```python
from build123d import *

# Parameters (mm, degrees)
SKETCH_1_R            = 7
EXTRUDE_1_DEPTH       = 10
SKETCH_9_W            = 7.120641766
SKETCH_9_H            = 4.534999238
EXTRUDE_6_DEPTH       = 1
SKETCH_11_W           = 1.257653538
SKETCH_11_H           = 9
EXTRUDE_7_DEPTH       = 4.5
EXTRUDE_8_DEPTH       = 6
FILLET_8_R            = 1
FILLET_9_R            = 1
CUT_EXTRUDE_1_DEPTH   = 10
SKETCH_14_W           = 1
SKETCH_14_H           = 3
EXTRUDE_9_DEPTH       = 3.122043073
SKETCH_15_W           = 1
SKETCH_15_H           = 3
EXTRUDE_10_DEPTH      = 4
EXTRUDE_11_DEPTH      = 0.2
EXTRUDE_11_DEPTH_BACK = 1.043632387
SKETCH_16_W           = 9.952294967
SKETCH_16_H           = 3.01746433
FILLET_11_R           = 1
FILLET_12_R           = 1
FILLET_13_R           = 1
FILLET_14_R           = 1
CUT_EXTRUDE_2_DEPTH   = 10
SKETCH_18_W           = 2.5
SKETCH_18_H           = 7.68123899
CUT_EXTRUDE_3_DEPTH   = 10
SKETCH_19_W           = 1.790352256
SKETCH_19_H           = 7.68123899
CUT_EXTRUDE_4_DEPTH   = 2
SKETCH_20_W           = 1.790352256
SKETCH_20_H           = 7.649055087
CUT_EXTRUDE_5_DEPTH   = 2
FILLET_15_R           = 1
FILLET_16_R           = 1
FILLET_17_R           = 1
FILLET_18_R           = 1


with BuildPart() as part:
    # Sketch 1 → Extrude 1 (new body)
    with BuildSketch(Plane(origin=(0.382706605, 0, 0), x_dir=(1, 0, 0), z_dir=(0, 0, 1))):
        with Locations((-75.594417438, 2.55)):
            Circle(SKETCH_1_R)
    extrude(amount=EXTRUDE_1_DEPTH)

    # Sketch 9 → Extrude 6 (add)
    with BuildSketch(Plane(origin=(6.127831546, 0, 9), x_dir=(1, 0, 0), z_dir=(0, 0, 1))):
        with Locations((-75.644850643, 2.267499619)):
            Rectangle(SKETCH_9_W, SKETCH_9_H)
    extrude(amount=EXTRUDE_6_DEPTH)



with BuildPart() as body_2:
    # Sketch 11 → Extrude 7 (new body)
    with BuildSketch(Plane(origin=(9.574526933, 4.534999238, 0.48426017), x_dir=(1, 0, 0), z_dir=(0, 1, 0))):
        with Locations((-76.184774061, -4.5)):
            Rectangle(SKETCH_11_W, SKETCH_11_H)
    extrude(amount=-EXTRUDE_7_DEPTH)


with BuildPart() as part_1:
    add(part.part)

    add(body_2.part)  # Extrude 8 merges body 2
    # Sketch 12 → Extrude 8 (add)
    with BuildSketch(Plane.ZY.offset(67.239073897)):
        Polygon((0.48426017, 4.534999238), (0.48426017, 0), (1.483647509, 0.034999238), (1.483647509, 4.534999238), align=None)
    extrude(amount=EXTRUDE_8_DEPTH)

    # Fillet 8
    fillet_8_edges = [part_1.edges().sort_by_distance(p)[0] for p in [
        (-65.981420359, 2.284999238, 0.48426017),
    ]]
    fillet(fillet_8_edges, radius=FILLET_8_R)

    # Fillet 9
    fillet_9_edges = [part_1.edges().sort_by_distance(p)[0] for p in [
        (-65.956698214, 2.267499619, 10),
    ]]
    fillet(fillet_9_edges, radius=FILLET_9_R - 0.0001)  # a hair under: the kernel refuses the full size

    # Sketch 13 → Cut-Extrude 1 (cut)
    with BuildSketch(Plane(origin=(0, 0, 0), x_dir=(-1, 0, 0), z_dir=(0, 0, -1))):
        with BuildLine():
            Line((69.812827514, 7.005564937), (69.812827514, -1.905564937))
            ThreePointArc((69.812827514, -1.905564937), (67.081734981, 2.55), (69.812827514, 7.005564937))
        make_face()
    extrude(amount=-CUT_EXTRUDE_1_DEPTH, mode=Mode.SUBTRACT)


with BuildPart() as cut_extrude_1_kept_piece:
    # of the separate pieces the step leaves, the one the design keeps (cut_extrude_1_pieces_kept)
    add(part_1.part.solids().sort_by_distance((-69.812827514, 7.005564937, 10))[0])

    # Sketch 14 → Extrude 9 (add)
    with BuildSketch(Plane(origin=(-69.812827514, 0, 0), x_dir=(0, 0, -1), z_dir=(1, 0, 0))):
        with Locations((-9.5, 2.417510407)):
            Rectangle(SKETCH_14_W, SKETCH_14_H)
    extrude(amount=EXTRUDE_9_DEPTH)

    # Sketch 15 → Extrude 10 (add)
    with BuildSketch(Plane(origin=(-69.812827514, 0, 0), x_dir=(0, 0, -1), z_dir=(1, 0, 0))):
        with Locations((-0.5, 2.417510407)):
            Rectangle(SKETCH_15_W, SKETCH_15_H)
    extrude(amount=EXTRUDE_10_DEPTH)

    # Sketch 16 → Extrude 11 (add, two sides: drawn at the far end of the back side and taken through both)
    with BuildSketch(Plane(origin=(-65.812827514, 0, 0), x_dir=(0, 0, -1), z_dir=(1, 0, 0)).offset(-EXTRUDE_11_DEPTH_BACK)):
        with Locations((-4.976147484, 2.408778242)):
            Rectangle(SKETCH_16_W, SKETCH_16_H)
    extrude(amount=EXTRUDE_11_DEPTH + EXTRUDE_11_DEPTH_BACK)

    # Fillet 11
    fillet_11_edges = [cut_extrude_1_kept_piece.edges().sort_by_distance(p)[0] for p in [
        (-65.612827514, 2.408778242, 0),
    ]]
    fillet(fillet_11_edges, radius=FILLET_11_R)

    # Fillet 12
    fillet_12_edges = [cut_extrude_1_kept_piece.edges().sort_by_distance(p)[0] for p in [
        (-65.612827514, 2.408778242, 9.952294967),
    ]]
    fillet(fillet_12_edges, radius=FILLET_12_R)

    # Fillet 13
    fillet_13_edges = [cut_extrude_1_kept_piece.edges().sort_by_distance(p)[0] for p in [
        (-69.812827514, 7.005564937, 5),
    ]]
    fillet(fillet_13_edges, radius=FILLET_13_R)

    # Fillet 14
    fillet_14_edges = [cut_extrude_1_kept_piece.edges().sort_by_distance(p)[0] for p in [
        (-69.812827514, -1.905564937, 5),
    ]]
    fillet(fillet_14_edges, radius=FILLET_14_R)

    # Sketch 17 → Cut-Extrude 2 (cut)
    with BuildSketch(Plane(origin=(0, 0, 0), x_dir=(-1, 0, 0), z_dir=(0, 0, -1))):
        with BuildLine():
            Line((80.617907093, 6.99668888), (80.617907093, -1.89668888))
            ThreePointArc((80.617907093, -1.89668888), (82.589637241, 2.55), (80.617907093, 6.99668888))
        make_face()
    extrude(amount=-CUT_EXTRUDE_2_DEPTH, mode=Mode.SUBTRACT)

    # Sketch 18 → Cut-Extrude 3 (cut)
    with BuildSketch(Plane(origin=(0, 0, 0), x_dir=(-1, 0, 0), z_dir=(0, 0, -1))):
        with Locations((77.577554837, 2.579171883)):
            Rectangle(SKETCH_18_W, SKETCH_18_H)
    extrude(amount=-CUT_EXTRUDE_3_DEPTH, mode=Mode.SUBTRACT)

    # Sketch 19 → Cut-Extrude 4 (cut)
    with BuildSketch(Plane(origin=(0, 0, 0), x_dir=(-1, 0, 0), z_dir=(0, 0, -1))):
        with Locations((79.722730965, 2.579171883)):
            Rectangle(SKETCH_19_W, SKETCH_19_H)
    extrude(amount=-CUT_EXTRUDE_4_DEPTH, mode=Mode.SUBTRACT)

    # Sketch 20 → Cut-Extrude 5 (cut)
    with BuildSketch(Plane.XY.offset(10)):
        with Locations((-79.722730965, 2.595263834)):
            Rectangle(SKETCH_20_W, SKETCH_20_H)
    extrude(amount=-CUT_EXTRUDE_5_DEPTH, mode=Mode.SUBTRACT)

    # Fillet 15
    fillet_15_edges = [cut_extrude_1_kept_piece.edges().sort_by_distance(p)[0] for p in [
        (-80.617907093, 6.708240129, 0),
    ]]
    fillet(fillet_15_edges, radius=FILLET_15_R)

    # Fillet 16
    fillet_16_edges = [cut_extrude_1_kept_piece.edges().sort_by_distance(p)[0] for p in [
        (-80.617907093, 6.708240129, 10),
    ]]
    fillet(fillet_16_edges, radius=FILLET_16_R)

    # Fillet 17
    fillet_17_edges = [cut_extrude_1_kept_piece.edges().sort_by_distance(p)[0] for p in [
        (-80.617907093, -1.579068246, 0),
    ]]
    fillet(fillet_17_edges, radius=FILLET_17_R)

    # Fillet 18
    fillet_18_edges = [cut_extrude_1_kept_piece.edges().sort_by_distance(p)[0] for p in [
        (-80.617907093, -1.562976295, 10),
    ]]
    fillet(fillet_18_edges, radius=FILLET_18_R)


solid = cut_extrude_1_kept_piece.part
```
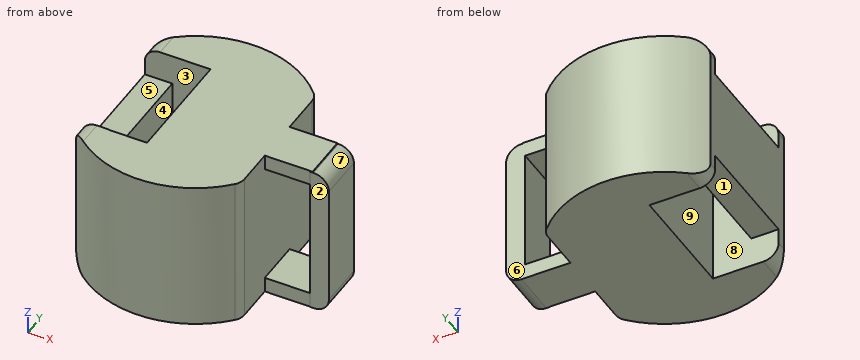
Design review of the part built by this model. Coordinates are the model's own, in mm. Face numbers are marked on the shaded views. A direction names the side the tool comes from. Give positions to 0.01 mm unless a question says otherwise; leave off trailing zeros. Write each loop counter-clockwise with the first axis right and the second up, starting at its lowest first coordinate (ties: lowest second). Pieces come first, ordered by that corner, then holes. Notation, with made-up numbers: (-18.75, 27) - (-0.75, 27) arc R25 cw to (-0.75, 40) - close; hole circle Ø10 at (-18.75, 0.25). An arc over 180 degrees is marked (long way). Return JSON: item names as keys, results as strings. Group by question number.
(1) Insertion check: pin 1 (0.6 mm diameter, centred on x = -66, z = 3.5, fed in from -Y); pin 2 (0.5 mm diameter, centred on x = -80, y = 3.5, fed in from +Z); pin 3 (1.5 mm diameter, centred on x = -77.5, z = 8, fed in from -Y). Each pin has a flat end and moves straight along its axis. Give the tip position at first contact, or say it passes through.
(2) We need section B-B, the plane y = -0.25. Give the boundary of the cut face in (x, z).
(3) We need section D-D, the plane z = 6. Give the boundary of the cut face in (x, y).
(4) To check wall thickness, follow probe 1 along X at (y, z) = (3.75, 7.75); probe 2 along X at (y, z) = (0.25, 7); probe 3 along Y at (x, z) = (-78.75, 2.5). State the ranges of each line that lie inside material, in increasing order.
(5) Machinability: for the marked faces 1, 2, 3, 4 and 5, which of the approach directions +Z, -Z, +X, -X, +Y, -Y give a long, thin tool a straight path to every point of the face, cutting with its end or side? Answer none if there is none.
(6) We need section C-C, the plane x = -68.5. Give the boundary of the cut face in (y, z).
(7) Mouldability with a two-part tool opening along Y and no side actions: class the marked faces 6, 7, 8 and 9 as +Y half, -Y half, draft (parallel to the pull), parting line (faces both ways), or undercut.
Reported:
{
 "1": {"pin 1": "stops at y = 0.9", "pin 2": "stops at z = 8", "pin 3": "stops at y = -4.28"},
 "2": {"outline": "(-80.62, 2) - (-78.83, 2) - (-78.83, 8) - (-80.62, 8) - close; (-76.33, 0) - (-69.81, 0) - (-69.81, 10) - (-76.33, 10) - close"},
 "3": {"outline": "(-80.62, -1.9) arc R7 ccw to (-70.08, -2.21) arc R1 ccw to (-69.81, -1.53) - (-69.81, 6.63) arc R1 ccw to (-70.08, 7.31) arc R7 ccw to (-80.62, 7) - close; (-66.86, 0.9) - (-65.61, 0.9) - (-65.61, 3.92) - (-66.86, 3.92) - close; hole (-78.83, -1.26) - (-76.33, -1.26) - (-76.33, 6.42) - (-78.83, 6.42) - close"},
 "4": {"probe 1": "x = -80.62 to -78.83, -76.33 to -69.81, -66.86 to -65.61", "probe 2": "x = -80.62 to -78.83, -76.33 to -69.81", "probe 3": "y = -3.49 to -1.26, 6.42 to 8.59"},
 "5": {"face 1": "-Z, -X", "face 2": "+Z, -Z, +X, -Y", "face 3": "none", "face 4": "+Z, -Z", "face 5": "+Z, -X"},
 "6": {"outline": "(0.92, 0) - (3.92, 0) - (3.92, 1) - (0.92, 1) - close; (0.92, 9) - (3.92, 9) - (3.92, 10) - (0.92, 10) - close"},
 "7": {"face 6": "+Y half", "face 7": "draft", "face 8": "undercut", "face 9": "undercut"}
}
